Check sheet for the modelled part. Datum: model origin and axes. Units: mm. A direction names the side the tool comes from. Give positions to 0.01 mm unless a question says otherwise; leave off trailing zeros. Loops run counter-clockwise (first coordinate to the right, second up) from the corner with the lowest first, then second, coordinate; pieces in that order, holes last.
```python
from build123d import *

# Parameters (mm, degrees)
REVOLUCI_N3_ANGLE       = 180
VACIADO1_T              = -2
CROQUIS5_R              = 60
CROQUIS5_R_2            = 58
SALIENTE_EXTRUIR1_DEPTH = 17.5
CROQUIS6_R              = 60
CROQUIS6_R_2            = 42
CROQUIS6_R_3            = 3
SALIENTE_EXTRUIR2_DEPTH = 6
CROQUIS7_R              = 24
CROQUIS7_R_2            = 22.5
SALIENTE_EXTRUIR3_DEPTH = 20
CROQUIS8_R              = 22.5
CORTAR_EXTRUIR2_DEPTH   = 20
CROQUIS9_R              = 22.5
CORTAR_EXTRUIR3_DEPTH   = 64.5
SALIENTE_EXTRUIR4_REACH = 65.5
CORTAR_EXTRUIR4_DEPTH   = 4


with BuildPart() as part:
    # Croquis4 → Revolución3 (revolve)
    with BuildSketch(Plane(origin=(0, 0, 0), x_dir=(0, 0, -1), z_dir=(1, 0, 0))):
        with BuildLine():
            Line((-60, 0), (60, 0))
            ThreePointArc((60, 0), (0, 60), (-60, 0))
        make_face()
    revolve(axis=Axis((0, 0, 60), (0, 0, 1)), revolution_arc=REVOLUCI_N3_ANGLE)

    # Vaciado1
    vaciado1_openings = [part.faces().sort_by_distance(p)[0] for p in [
        (0, 0, -60),
    ]]
    offset(amount=VACIADO1_T, openings=vaciado1_openings)

    # Croquis5 → Saliente-Extruir1 (add)
    with BuildSketch(Plane(origin=(0, 0, 0), x_dir=(0, 0, -1), z_dir=(1, 0, 0))):
        Circle(CROQUIS5_R)
        Circle(CROQUIS5_R_2, mode=Mode.SUBTRACT)
    extrude(amount=SALIENTE_EXTRUIR1_DEPTH)

    # Croquis6 → Saliente-Extruir2 (add)
    with BuildSketch(Plane(origin=(17.5, 0, 0), x_dir=(0, 0, -1), z_dir=(1, 0, 0))):
        Circle(CROQUIS6_R)
        Circle(CROQUIS6_R_2, mode=Mode.SUBTRACT)
        with Locations((0, 51)):
            Circle(CROQUIS6_R_3, mode=Mode.SUBTRACT)
        with Locations((44.167295593, 25.5)):
            Circle(CROQUIS6_R_3, mode=Mode.SUBTRACT)
        with Locations((44.167295593, -25.5)):
            Circle(CROQUIS6_R_3, mode=Mode.SUBTRACT)
        with Locations((0, -51)):
            Circle(CROQUIS6_R_3, mode=Mode.SUBTRACT)
        with Locations((-44.167295593, -25.5)):
            Circle(CROQUIS6_R_3, mode=Mode.SUBTRACT)
        with Locations((-44.167295593, 25.5)):
            Circle(CROQUIS6_R_3, mode=Mode.SUBTRACT)
    extrude(amount=SALIENTE_EXTRUIR2_DEPTH)

    # Croquis7 → Saliente-Extruir3 (add)
    with BuildSketch(Plane(origin=(23.5, 0, 0), x_dir=(0, 0, -1), z_dir=(1, 0, 0))):
        with Locations((59.439232835, -51)):
            Circle(CROQUIS7_R)
        with Locations((59.439232835, -51)):
            Circle(CROQUIS7_R_2, mode=Mode.SUBTRACT)
        with Locations((-59.439232835, -51)):
            Circle(CROQUIS7_R)
        with Locations((-59.439232835, -51)):
            Circle(CROQUIS7_R_2, mode=Mode.SUBTRACT)
    extrude(amount=-SALIENTE_EXTRUIR3_DEPTH)

    # Croquis8 → Cortar-Extruir2 (cut)
    with BuildSketch(Plane(origin=(23.5, 0, 0), x_dir=(0, 0, -1), z_dir=(1, 0, 0))):
        with Locations((-59.439232835, -51)):
            Circle(CROQUIS8_R)
        with Locations((59.439232835, -51)):
            Circle(CROQUIS8_R)
    extrude(amount=-CORTAR_EXTRUIR2_DEPTH, mode=Mode.SUBTRACT)

    # Croquis9 → Cortar-Extruir3 (cut, through all)
    with BuildSketch(Plane(origin=(3.5, 0, 0), x_dir=(0, 0, -1), z_dir=(1, 0, 0))):
        with Locations((-59.439232835, -51)):
            Circle(CROQUIS9_R)
        with Locations((59.439232835, -51)):
            Circle(CROQUIS9_R)
    extrude(amount=-CORTAR_EXTRUIR3_DEPTH, mode=Mode.SUBTRACT)

    # Croquis10 → Saliente-Extruir4 (add, up to next)
    with BuildSketch(Plane(origin=(3.5, 0, 0), x_dir=(0, 0, -1), z_dir=(1, 0, 0)), mode=Mode.PRIVATE) as saliente_extruir4_sk1:
        with BuildLine():
            ThreePointArc((-37.297899218, -46.998582041), (-42.363355169, -36.348569969), (-52.120051429, -29.723731917))
            ThreePointArc((-52.120051429, -29.723731917), (-52.804439439, -28.490194375), (-53.459638302, -27.240908072))
            ThreePointArc((-53.459638302, -27.240908072), (-40.845499377, -35.046220633), (-35.047443828, -48.699863256))
            ThreePointArc((-35.047443828, -48.699863256), (-36.182672021, -47.86245131), (-37.297899218, -46.998582041))
        make_face()
    saliente_extruir4_tool1 = extrude(saliente_extruir4_sk1.sketch, amount=-SALIENTE_EXTRUIR4_REACH, mode=Mode.PRIVATE) - part.part
    add(saliente_extruir4_tool1.solids().sort_by_distance((3.5, -28.355933, 52.555595))[0])
    # Croquis10 → Saliente-Extruir4 (add, up to next)
    with BuildSketch(Plane(origin=(3.5, 0, 0), x_dir=(0, 0, -1), z_dir=(1, 0, 0)), mode=Mode.PRIVATE) as saliente_extruir4_sk2:
        with BuildLine():
            ThreePointArc((37.297899218, -46.998582041), (36.182672021, -47.86245131), (35.047443828, -48.699863256))
            ThreePointArc((35.047443828, -48.699863256), (40.845499377, -35.046220633), (53.459638302, -27.240908072))
            ThreePointArc((53.459638302, -27.240908072), (52.804439439, -28.490194375), (52.120051429, -29.723731917))
            ThreePointArc((52.120051429, -29.723731917), (42.363355169, -36.348569969), (37.297899218, -46.998582041))
        make_face()
    saliente_extruir4_tool2 = extrude(saliente_extruir4_sk2.sketch, amount=-SALIENTE_EXTRUIR4_REACH, mode=Mode.PRIVATE) - part.part
    add(saliente_extruir4_tool2.solids().sort_by_distance((3.5, -36.164448, -42.148766))[0])

    # Croquis11 → Cortar-Extruir4 (cut)
    with BuildSketch(Plane.ZY.offset(-17.5)):
        Polygon((48.167295593, 27.809401077), (44.167295593, 30.118802154), (40.167295593, 27.809401077), (40.167295593, 23.190598923), (44.167295593, 20.881197846), (48.167295593, 23.190598923), align=None)
        Polygon((0, 55.618802154), (-4, 53.309401077), (-4, 48.690598923), (0, 46.381197846), (4, 48.690598923), (4, 53.309401077), align=None)
        Polygon((48.167295593, -27.809401077), (48.167295593, -23.190598923), (44.167295593, -20.881197846), (40.167295593, -23.190598923), (40.167295593, -27.809401077), (44.167295593, -30.118802154), align=None)
        Polygon((0, -55.618802154), (4, -53.309401077), (4, -48.690598923), (0, -46.381197846), (-4, -48.690598923), (-4, -53.309401077), align=None)
        Polygon((-48.167295593, -27.809401077), (-44.167295593, -30.118802154), (-40.167295593, -27.809401077), (-40.167295593, -23.190598923), (-44.167295593, -20.881197846), (-48.167295593, -23.190598923), align=None)
        Polygon((-48.167295593, 27.809401077), (-48.167295593, 23.190598923), (-44.167295593, 20.881197846), (-40.167295593, 23.190598923), (-40.167295593, 27.809401077), (-44.167295593, 30.118802154), align=None)
    extrude(amount=-CORTAR_EXTRUIR4_DEPTH, mode=Mode.SUBTRACT)


solid = part.part
```
(1) Material ranges on line 1 (Z direction, x = 22, y = -51); line 2 (X direction, y = -28.5, z = 57.5); line 3 (Z direction, x = -34, y = 14), recorded low to high.
(2) Section check D-D on y = -51. Give the number of separate pieces and of enclosed holes in the cut face, plus the area to 3 significant figures.
(3) Release check for a two-part mould opening along X. For faces 3 (the face through (19, 25, 48.167)), 4 (the face through (22, -48, 0)), 5 (the face through (3.5, -67, 76)) record: pulls with the +X half, pulls with the -X half, needs draft (parallel to the pull), parting line crosses it, or undercut.
(4) Gauge pin test, flat ends, axial feed: pin 1 Ø8 at (x, z) = (12.5, -16.5) entering from -Y; pin 2 Ø9 at (y, z) = (-25.5, 43) entering from -X; pin 3 Ø4 at (x, z) = (-13.5, -1.5) entering from -Y; pin 4 Ø24 at (y, z) = (-51.5, -51.5) entering from -X. Record the tip position at first contact, or that the pin passes through.
(5) Section check A-A on y = 25.5. Record the boundary of the cut face in (x, z).
(6) Section check C-C on z = 64.5. Record the boundary of the cut face in (x, y).
(7) Section check B-B on y = 0. Record the boundary of the cut face in (x, z), plus the area to 3 significant figures.
(8) Access from +Z, -Z, +X, -X, +Y, -Y to the whole of each face (thin tool, end or side, straight path). Record for faces 1 (the face through (20.46, 12.62, -40.06)), 2 (the face through (19.47, -22.02, -46.14)).
Computed values:
1. line 1: z = -83.44 to -81.94, -36.94 to -35.44, -31.61 to -3, 3 to 31.61, 35.44 to 36.94, 81.94 to 83.44
1. line 2: x = 3.5 to 23.5
1. line 3: z = -47.41 to -44.86, 44.86 to 47.41
2. separate pieces: 5
2. enclosed holes: 0
2. area: 965 mm2
3. face 3: undercut
3. face 4: needs draft
3. face 5: pulls with the -X half
4. pin 1: stops at y = -58.68
4. pin 2: stops at x = -39.12
4. pin 3: stops at y = -58.87
4. pin 4: passes through
5. outline: (0, -54.31) - (23.5, -54.31) - (23.5, -47.17) - (21.5, -47.17) - (21.5, -48.17) - (17.5, -48.17) - (17.5, -52.09) - (0, -52.09) arc R52.09 cw to (0, 52.09) - (17.5, 52.09) - (17.5, 48.17) - (21.5, 48.17) - (21.5, 47.17) - (23.5, 47.17) - (23.5, 54.31) - (0, 54.31) arc R54.31 ccw to start; (17.5, -40.17) - (21.5, -40.17) - (21.5, -41.17) - (23.5, -41.17) - (23.5, -33.37) - (17.5, -33.37) - close; (17.5, 33.37) - (23.5, 33.37) - (23.5, 41.17) - (21.5, 41.17) - (21.5, 40.17) - (17.5, 40.17) - close
6. outline: (3.5, -74.46) - (23.5, -74.46) - (23.5, -72.92) - (3.5, -72.92) - close; (3.5, -29.08) - (23.5, -29.08) - (23.5, -27.54) - (3.5, -27.54) - close
7. outline: (0, -60) - (23.5, -60) - (23.5, -42) - (17.5, -42) - (17.5, -58) - (0, -58) arc R58 cw to (0, 58) - (17.5, 58) - (17.5, 42) - (23.5, 42) - (23.5, 60) - (0, 60) arc R60 ccw to start
7. area: 657 mm2
8. face 1: +X
8. face 2: none
